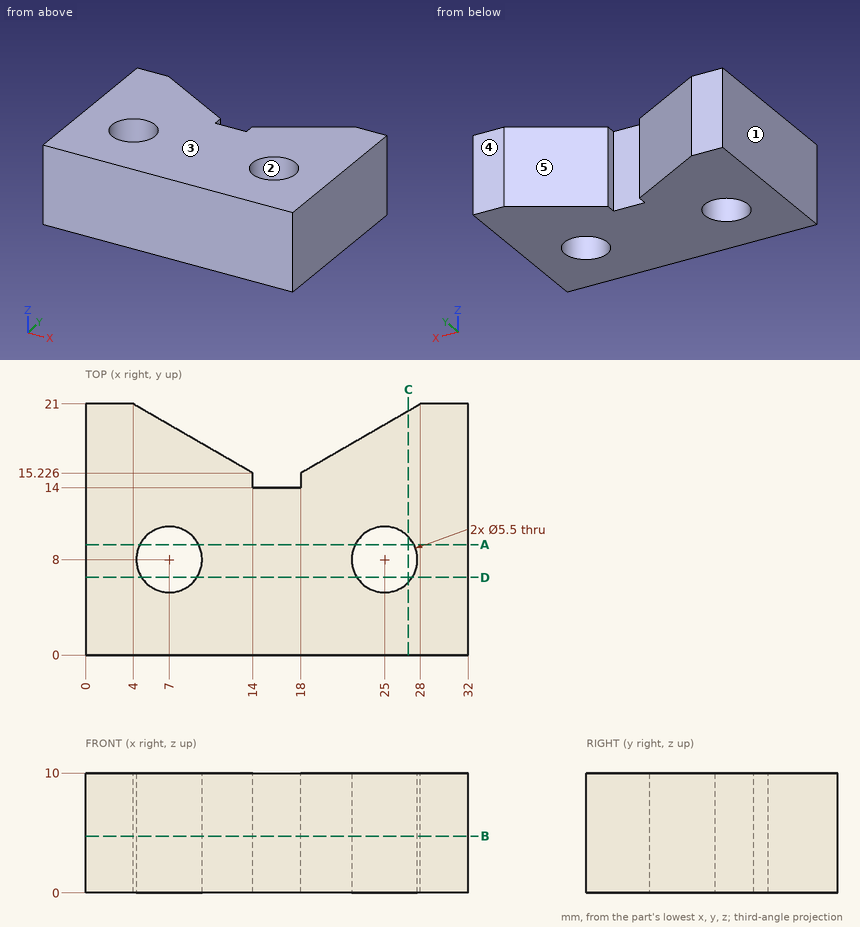
Verification items for this drawing (mm, ordinates from the low corner). A direction names the side the tool comes from. Give positions to 0.01 mm unless a question says otherwise; leave off trailing zeros. Loops run counter-clockwise (first coordinate to the right, second up) from the corner with the lowest first, then second, coordinate; pieces in that order, holes last. Notation, with made-up numbers: M 41.5,58 L 51.5,58 A32 ccw 51.5,90 Z; hole C 48,86.25 d9. An arc over 180 degrees is marked long. Return JSON: item names as keys, results as strings. Group by question number.
1. Thickness scan on L1, parallel to X at y = 14.25, z = 1; L2, parallel to X at y = 7.75, z = 1; L3, parallel to X at y = 6.5, z = 7.25 (1 decimal). Record the ranges inside material, lowest first.
2. Go/stop test with flat-tipped pins: pin 1 (4.5 mm diameter, centred on x = 15.5, z = 5, fed in from +Y); pin 2 (1 mm diameter, centred on x = 9.5, z = 8, fed in from +Y). Record where each tip stops, or that it passes through.
3. Cross-section at C-C on x = 27. Record the boundary of the cut face in (y, z).
4. Tool access check on the marked faces 4 and 5. Record the directions out of +Z, -Z, +X, -X, +Y, -Y that give a thin tool (end or side, any length) a straight path to the whole face; none if there is none.
5. Cross-section at B-B on z = 4.75. Record the boundary of the cut face in (x, y).
6. Cross-section at A-A on y = 9.25. Record the boundary of the cut face in (x, z), plus the area to 3 significant figures.
7. Cross-section at D-D on y = 6.5. Record the boundary of the cut face in (x, z) (1 decimal).
8. Mould release check, pull along X, two halves, no side actions. Record for the marked faces 1, 2 and 3: released by +X, released by -X, zero draft, split by the parting line, or undercut.
Return value:
{
 "1": {"L1": "0 to 14, 18 to 32", "L2": "0 to 4.26, 9.74 to 22.26, 27.74 to 32", "L3": "0 to 4.7, 9.3 to 22.7, 27.3 to 32"},
 "2": {"pin 1": "y = 15.66", "pin 2": "y = 18.11"},
 "3": {"outline": "M 0,0 L 6.11,0 L 6.11,10 L 0,10 Z; M 9.89,0 L 20.42,0 L 20.42,10 L 9.89,10 Z"},
 "4": {"face 4": "+Z, -Z, +X, -X, +Y", "face 5": "+Z, -Z, +Y"},
 "5": {"outline": "M 0,0 L 32,0 L 32,21 L 28,21 L 18,15.23 L 18,14 L 14,14 L 14,15.23 L 4,21 L 0,21 Z; hole C 7,8 d5.5; hole C 25,8 d5.5"},
 "6": {"outline": "M 0,0 L 4.55,0 L 4.55,10 L 0,10 Z; M 9.45,0 L 22.55,0 L 22.55,10 L 9.45,10 Z; M 27.45,0 L 32,0 L 32,10 L 27.45,10 Z", "area": "222 mm^2"},
 "7": {"outline": "M 0,0 L 4.7,0 L 4.7,10 L 0,10 Z; M 9.3,0 L 22.7,0 L 22.7,10 L 9.3,10 Z; M 27.3,0 L 32,0 L 32,10 L 27.3,10 Z"},
 "8": {"face 1": "released by -X", "face 2": "undercut", "face 3": "zero draft"}
}
